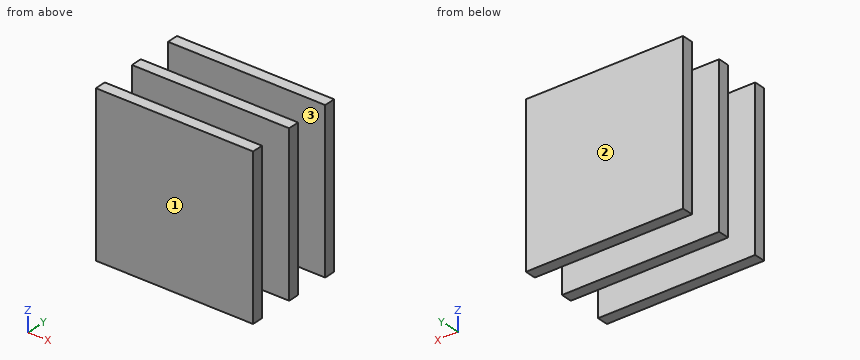
from build123d import *

# Parameters (mm, degrees)
ESQUISSE1_W      = 250
ESQUISSE1_H      = 250
EXTRUSION1_DEPTH = 18
ESQUISSE2_W      = 70
ESQUISSE2_H      = 70
EXTRUSION2_DEPTH = 54.5
ESQUISSE3_W      = 250
ESQUISSE3_H      = 250
EXTRUSION3_DEPTH = 18
ESQUISSE4_W      = 70
ESQUISSE4_H      = 70
EXTRUSION4_DEPTH = 54.5
ESQUISSE5_W      = 250
ESQUISSE5_H      = 250
EXTRUSION5_DEPTH = 18


with BuildPart() as part:
    # Esquisse1 → Extrusion1 (new body)
    with BuildSketch(Plane(origin=(0, 0, 0), x_dir=(1, 0, 0), z_dir=(0, 1, 0))):
        with Locations((125, 125)):
            Rectangle(ESQUISSE1_W, ESQUISSE1_H)
    extrude(amount=EXTRUSION1_DEPTH)

    # Esquisse2 → Extrusion2 (add)
    with BuildSketch(Plane(origin=(0, 18, 0), x_dir=(-1, 0, 0), z_dir=(0, 1, 0))):
        with Locations((-125, -125)):
            Rectangle(ESQUISSE2_W, ESQUISSE2_H)
    extrude(amount=EXTRUSION2_DEPTH)

    # Esquisse3 → Extrusion3 (add)
    with BuildSketch(Plane(origin=(0, 72.5, 0), x_dir=(1, 0, 0), z_dir=(0, 1, 0))):
        with Locations((125, 125)):
            Rectangle(ESQUISSE3_W, ESQUISSE3_H)
    extrude(amount=EXTRUSION3_DEPTH)

    # Esquisse4 → Extrusion4 (add)
    with BuildSketch(Plane(origin=(0, 90.5, 0), x_dir=(1, 0, 0), z_dir=(0, 1, 0))):
        with Locations((125, 125)):
            Rectangle(ESQUISSE4_W, ESQUISSE4_H)
    extrude(amount=EXTRUSION4_DEPTH)

    # Esquisse5 → Extrusion5 (add)
    with BuildSketch(Plane(origin=(0, 145, 0), x_dir=(1, 0, 0), z_dir=(0, 1, 0))):
        with Locations((125, 125)):
            Rectangle(ESQUISSE5_W, ESQUISSE5_H)
    extrude(amount=EXTRUSION5_DEPTH)


solid = part.part
Source: CAD feature listing. Evaluate the final solid. Frame: model axes, mm. Face numbers are marked on the shaded views. Round coordinates to 2 decimals unless told otherwise and drop trailing zeros. Order: outer loops, then holes, each group sorted by start corner. A loop starts at its lowest first (then second) coordinate and runs counter-clockwise, first axis right, second up. Notation, with made-up numbers: (-27.75, -12) - (25.25, -12) arc R12 ccw to (25.25, 2) - close; hole circle Ø5 at (6.5, 36.5). An arc over 180 degrees is marked (long way). Use a Markdown table: item, result. Add a question column.
1. Section query D-D (x = 128.5). Return the cut outline in (y, z), then the cut area to 3 significant figures.
2. First-contact query: pin 1 (8 mm diameter, centred on x = 130, y = 125, fed in from +Z); pin 2 (16.5 mm diameter, centred on x = 141, y = 42, fed in from -Z); pin 3 (1 mm diameter, centred on y = 117.5, z = -143.5, fed in from -X). Flat tips, straight axial feed; report the tip coordinate or a pass-through.
3. Line query: probe 1 along Y at (x, z) = (169.5, -169); probe 2 along X at (y, z) = (141, -136); probe 3 along Z at (x, y) = (128, 37). Output: solid intervals per line, ascending.
4. Mould query, pull axis Y, two halves, no side actions, for the marked faces 1, 2 and 3. Classes: +Y half, -Y half, draft (parallel to the pull), parting line (faces both ways), or undercut.
5. Section query B-B (z = -29). Return the cut outline in (x, y).
6. Section query C-C (z = -96). Return the cut outline in (x, y).
7. Section query A-A (x = 45). Return the cut outline in (y, z), then the cut area to 3 significant figures.
Derived:
| question | item | result |
|---|---|---|
| 1 | outline | (0, -250) - (18, -250) - (18, -160) - (72.5, -160) - (72.5, -250) - (90.5, -250) - (90.5, -160) - (145, -160) - (145, -250) - (163, -250) - (163, 0) - (145, 0) - (145, -90) - (90.5, -90) - (90.5, 0) - (72.5, 0) - (72.5, -90) - (18, -90) - (18, 0) - (0, 0) - close |
| 1 | area | 21,100 mm2 |
| 2 | pin 1 | z = -90 |
| 2 | pin 2 | z = -160 |
| 2 | pin 3 | x = 90 |
| 3 | probe 1 | 0 to 18, 72.5 to 90.5, 145 to 163 |
| 3 | probe 2 | 90 to 160 |
| 3 | probe 3 | -160 to -90 |
| 4 | face 1 | -Y half |
| 4 | face 2 | +Y half |
| 4 | face 3 | undercut |
| 5 | outline | (0, 0) - (250, 0) - (250, 18) - (0, 18) - close; (0, 72.5) - (250, 72.5) - (250, 90.5) - (0, 90.5) - close; (0, 145) - (250, 145) - (250, 163) - (0, 163) - close |
| 6 | outline | (0, 0) - (250, 0) - (250, 18) - (160, 18) - (160, 72.5) - (250, 72.5) - (250, 90.5) - (160, 90.5) - (160, 145) - (250, 145) - (250, 163) - (0, 163) - (0, 145) - (90, 145) - (90, 90.5) - (0, 90.5) - (0, 72.5) - (90, 72.5) - (90, 18) - (0, 18) - close |
| 7 | outline | (0, -250) - (18, -250) - (18, 0) - (0, 0) - close; (72.5, -250) - (90.5, -250) - (90.5, 0) - (72.5, 0) - close; (145, -250) - (163, -250) - (163, 0) - (145, 0) - close |
| 7 | area | 13,500 mm2 |
